Design review of the part built by this model. Coordinates are the model's own, in mm. Face numbers are marked on the shaded views. Round coordinates to 2 decimals unless told otherwise and drop trailing zeros. Loops run counter-clockwise (first coordinate to the right, second up) from the corner with the lowest first, then second, coordinate; pieces in that order, holes last. Notation, with made-up numbers: M 83.25,25 L 110.25,25 A19 ccw 110.25,39 Z; hole C 33.5,37 d4. An arc over 180 degrees is marked long. One line per item, written item: value. Start each with the question number.
Item 1: Mouldability with a two-part tool opening along X and no side actions: class the marked faces 1, 2 and 3 as released by +X, released by -X, zero draft, split by the parting line, or undercut.
Item 2: Clearance check with flat-ended pins moving along their axes: pin 1 (10 mm diameter, centred on y = -19, z = 16, fed in from +X); pin 2 (8 mm diameter, centred on x = 44, y = -3, fed in from -Z). State where each tip first meets the part, or that it passes through.
Item 3: We need section B-B (x = 0). Write out the cut boundary in (y, z), then the cut area to 3 significant figures.
Item 4: For line 1 along Z through (x, y) = (0, -17); line 2 along Z through (x, y) = (-2, -19.5); line 3 along X through (y, z) = (-17.75, -4.5), list the stretches that pass through material, from the lowest coordinate up.
Item 5: We need section C-C (z = 2.5). Write out the cut boundary in (x, y).
Item 6: We need section A-A (y = -13.25). Write out the cut boundary in (x, z), then the cut area to 3 significant figures.
Item 7: We need section D-D (x = 50.5). Write out the cut boundary in (y, z).
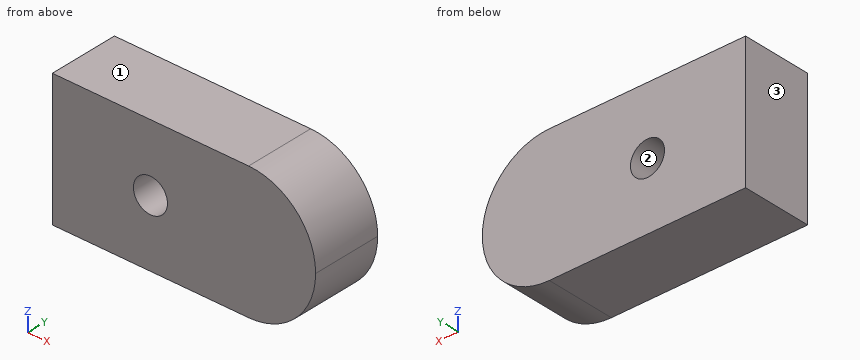
from build123d import *

# Parameters (mm, degrees)
F0_R     = 6.189108
F1_DEPTH = 25.4


with BuildPart() as f1:
    # F0 (on Front) → F1 (new body)
    with BuildSketch(Plane.XZ):
        with BuildLine():
            ThreePointArc((35.654567, -24.347987), (11.30658, 0), (35.654567, 24.347987))
            Line((35.654567, 24.347987), (-35.654567, 24.347987))
            Line((-35.654567, 24.347987), (-35.654567, -24.347987))
            Line((-35.654567, -24.347987), (35.654567, -24.347987))
        make_face()
        Circle(F0_R, mode=Mode.SUBTRACT)
        with BuildLine():
            Line((35.654567, -24.347987), (35.654567, 24.347987))
            ThreePointArc((35.654567, 24.347987), (11.30658, 0), (35.654567, -24.347987))
        make_face()
        with BuildLine():
            ThreePointArc((60.002554, 0), (52.871194, 17.216627), (35.654567, 24.347987))
            Line((35.654567, 24.347987), (35.654567, -24.347987))
            ThreePointArc((35.654567, -24.347987), (52.871194, -17.216627), (60.002554, 0))
        make_face()
    extrude(amount=F1_DEPTH)


solid = f1.part
A:
1. face 1: zero draft
1. face 2: undercut
1. face 3: released by -X
2. pin 1: x = 57.38
2. pin 2: z = -23.96
3. outline: M -25.4,-24.35 L 0,-24.35 L 0,-6.19 L -25.4,-6.19 Z; M -25.4,6.19 L 0,6.19 L 0,24.35 L -25.4,24.35 Z
3. area: 922 mm2
4. line 1: -24.35 to -6.19, 6.19 to 24.35
4. line 2: -24.35 to -5.86, 5.86 to 24.35
4. line 3: -35.65 to -4.25, 4.25 to 59.58
5. outline: M -35.65,-25.4 L -5.66,-25.4 L -5.66,0 L -35.65,0 Z; M 5.66,-25.4 L 59.87,-25.4 L 59.87,0 L 5.66,0 Z
6. outline: M -35.65,-24.35 L 35.65,-24.35 A24.35 ccw 60,0 A24.35 ccw 35.65,24.35 L -35.65,24.35 Z; hole C 0,0 d12.38
6. area: 4,280 mm2
7. outline: M -25.4,-19.3 L 0,-19.3 L 0,19.3 L -25.4,19.3 Z
